Input: part model. Units: mm. Frame: model coordinates. Face numbers are marked on the shaded views. A direction names the side the tool comes from. Coordinates: 2 decimals unless noted, no trailing zeros. Loops run counter-clockwise (first coordinate to the right, second up) from the corner with the lowest first, then second, coordinate; pieces in that order, holes last. Notation, with made-up numbers: M -1.5,15.25 L 54.5,15.25 A17 ccw 54.5,46.25 Z; hole C 64.5,31 d10. An arc over 180 degrees is marked long. Use a Markdown table: item, result. Add a question column.
1. Draft query along Y for the marked faces 3, 4 and 5. Return one class per face: +Y half, -Y half, draft (parallel to the pull), parting line (faces both ways), or undercut.
2. Section C-C on z = 3.25. Output: boundary loops of the cut face in (x, y), then the cut area to 3 significant figures.
3. Section D-D on y = -18. Output: boundary loops of the cut face in (x, z).
4. Section B-B on y = 3. Output: boundary loops of the cut face in (x, z), then the cut area to 3 significant figures.
5. Line query: L1, parallel to Y at x = 0, z = 4.5; L2, parallel to Z at x = 6.5, y = 22. Output: solid intervals per line, ascending. Write a range as [from, to].
6. Set-up query: the marked faces 1 and 2. Return all of +Z, -Z, +X, -X, +Y, -Y with unobstructed straight access to the full face (end or side cutting, diameter ignored); none if empty.
7. Pin query (flat end, axial travel): pin 1 (4 mm diameter, centred on x = -7.5, z = 9, fed in from -Y); pin 2 (4 mm diameter, centred on x = 0.5, z = 12.5, fed in from -Y); pin 3 (4 mm diameter, centred on y = -7, z = 10.5, fed in from -X). Return the tip coordinate at first contact, or that it passes through.
8. Section A-A on x = 0. Output: boundary loops of the cut face in (y, z).
```python
from build123d import *

# Parameters (mm, degrees)
F0_R     = 29
F1_DEPTH = 14
F2_W     = 29.5
F2_H     = 29.5
F3_DEPTH = 25
F4_R     = 26.5
F5_DEPTH = 9


with BuildPart() as f1:
    # F0 (on Top) → F1 (new body)
    with BuildSketch(Plane.XY):
        Circle(F0_R)
    extrude(amount=F1_DEPTH)

    # F2 (on face) → F3 (cut)
    with BuildSketch(Plane.XY.offset(14)):
        Rectangle(F2_W, F2_H)
    extrude(amount=-F3_DEPTH, mode=Mode.SUBTRACT)

    # F4 (on face) → F5 (cut)
    with BuildSketch(Plane(origin=(0, 0, 0), x_dir=(1, 0, 0), z_dir=(0, 0, -1))):
        Circle(F4_R)
    extrude(amount=-F5_DEPTH, mode=Mode.SUBTRACT)


solid = f1.part
```
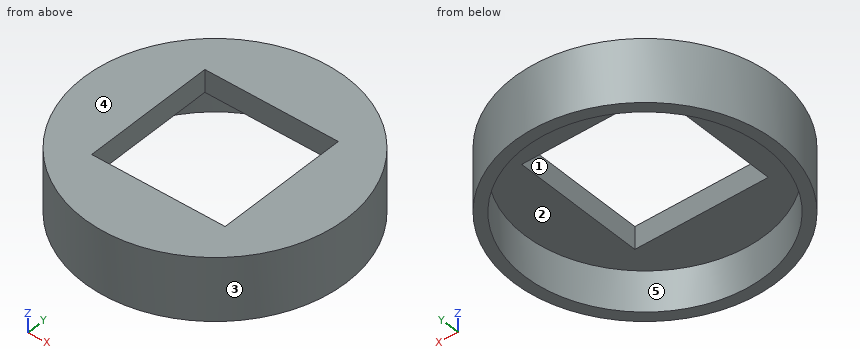
Answers below:
| question | item | result |
|---|---|---|
| 1 | face 3 | parting line |
| 1 | face 4 | draft |
| 1 | face 5 | undercut |
| 2 | outline | C 0,0 d58; hole C 0,0 d53 |
| 2 | area | 436 mm² |
| 3 | outline | M -22.74,0 L -19.45,0 L -19.45,9 L 19.45,9 L 19.45,0 L 22.74,0 L 22.74,14 L -22.74,14 Z |
| 4 | outline | M -28.84,0 L -26.33,0 L -26.33,9 L -14.75,9 L -14.75,14 L -28.84,14 Z; M 14.75,9 L 26.33,9 L 26.33,0 L 28.84,0 L 28.84,14 L 14.75,14 Z |
| 4 | area | 186 mm² |
| 5 | L1 | y = [-29, -26.5], [26.5, 29] |
| 5 | L2 | z = [9, 14] |
| 6 | face 1 | +Z, -Z |
| 6 | face 2 | -Z |
| 7 | pin 1 | stops at y = -28.47 |
| 7 | pin 2 | stops at y = -29 |
| 7 | pin 3 | stops at x = -28.57 |
| 8 | outline | M -29,0 L -26.5,0 L -26.5,9 L -14.75,9 L -14.75,14 L -29,14 Z; M 14.75,9 L 26.5,9 L 26.5,0 L 29,0 L 29,14 L 14.75,14 Z |
